For this review, take the finished solid that the model builds, in its own axes (mm). A direction names the side the tool comes from. Give positions to 0.01 mm unless a question says otherwise; leave off trailing zeros. Loops run counter-clockwise (first coordinate to the right, second up) from the corner with the lowest first, then second, coordinate; pieces in that order, holes last. Notation, with made-up numbers: (-22, -17.75) -> (-2, -17.75) arc R18 ccw to (-2, 9.25) -> close; hole circle Ø3 at (13.5, 10). An arc over 180 degrees is marked (long way). Write each question's results on one line, items separated by ' | '. Start each with the question number.
```python
from build123d import *

# Parameters (mm, degrees)
A_BASE_T42_OUTLINE_R               = 2.2479
A_BASE_T42_OUTLINE_R_2             = 1
A_BASE_T42_DEPTH                   = 3
OUTER_BRIM_DEPTH                   = 3
SKETCH5_W                          = 15
SKETCH5_H                          = 3
BASE_SUPPORTS_DEPTH                = 3
BASE_SUPPORTS_CHAMFER_SIZE         = 3
COVER_START                        = -3
SKETCH6_R                          = 1
COVER_DEPTH                        = 3
SKETCH2_W                          = 10.5
SKETCH2_H                          = 45
DYNAMIXEL_OFFSET_DEPTH             = 1.25
SKETCH3_W                          = 3
SKETCH3_H                          = 45
SKETCH3_H_2                        = 22.5
DYNAMIXEL_SIDE_SUPPORT_WALLS_DEPTH = 5.6
DYNAMIXEL_SUPPORT_CONTOURING_R     = 1


# Read off the part's stored shape, not the designer's step: a_base_t42
with BuildPart() as part:
    # a_base_t42 outline → a_base_t42 (new body)
    with BuildSketch(Plane(origin=(0, 0, 0), x_dir=(1, 0, 0), z_dir=(0, 1, 0))):
        with BuildLine():
            ThreePointArc((31.5, -42), (52.5, 0), (31.5, 42))
            Line((31.5, 42), (-31.5, 42))
            ThreePointArc((-31.5, 42), (-52.5, 0), (-31.5, -42))
            Line((-31.5, -42), (31.5, -42))
        make_face()
        with Locations((-23, -35)):
            Circle(A_BASE_T42_OUTLINE_R, mode=Mode.SUBTRACT)
        with Locations((23, -35)):
            Circle(A_BASE_T42_OUTLINE_R, mode=Mode.SUBTRACT)
        with Locations((-40.25, 0)):
            Circle(A_BASE_T42_OUTLINE_R_2, mode=Mode.SUBTRACT)
        with Locations((-23, 35)):
            Circle(A_BASE_T42_OUTLINE_R, mode=Mode.SUBTRACT)
        with Locations((40.25, 0)):
            Circle(A_BASE_T42_OUTLINE_R_2, mode=Mode.SUBTRACT)
        with Locations((23, 35)):
            Circle(A_BASE_T42_OUTLINE_R, mode=Mode.SUBTRACT)
    extrude(amount=A_BASE_T42_DEPTH)

    # Sketch1 → Outer Brim (add)
    with BuildSketch(Plane(origin=(0, 3, 0), x_dir=(1, 0, 0), z_dir=(0, 1, 0))):
        with BuildLine():
            Line((-31.5, -42), (31.5, -42))
            ThreePointArc((31.5, -42), (52.5, 0), (31.5, 42))
            Line((31.5, 42), (-31.5, 42))
            ThreePointArc((-31.5, 42), (-52.5, 0), (-31.5, -42))
        make_face()
        with BuildLine():
            Line((30.483602149, 39), (-30.483602149, 39))
            ThreePointArc((-30.483602149, 39), (-49.5, 0), (-30.483602149, -39))
            Line((-30.483602149, -39), (30.483602149, -39))
            ThreePointArc((30.483602149, -39), (49.5, 0), (30.483602149, 39))
        make_face(mode=Mode.SUBTRACT)
    extrude(amount=OUTER_BRIM_DEPTH)

    # Sketch5 → Base Supports (add)
    with BuildSketch(Plane(origin=(0, 3, 0), x_dir=(1, 0, 0), z_dir=(0, 1, 0))):
        with Locations((0, -27)):
            Rectangle(SKETCH5_W, SKETCH5_H)
        with Locations((0, 27)):
            Rectangle(SKETCH5_W, SKETCH5_H)
    extrude(amount=BASE_SUPPORTS_DEPTH)

    # Base Supports Chamfer
    base_supports_chamfer_edges = [part.edges().sort_by_distance(p)[0] for p in [
        (0, 3, 28.5),
        (0, 3, -28.5),
    ]]
    chamfer(base_supports_chamfer_edges, length=BASE_SUPPORTS_CHAMFER_SIZE - 0.0001)  # a hair under: the kernel refuses the full size

    # Sketch6 → Cover (add)
    with BuildSketch(Plane(origin=(0, 3, 0), x_dir=(1, 0, 0), z_dir=(0, 1, 0)).offset(COVER_START)):
        with Locations((-40.25, 0)):
            Circle(SKETCH6_R)
        with Locations((40.25, 0)):
            Circle(SKETCH6_R)
    extrude(amount=COVER_DEPTH)

    # Sketch2 → Dynamixel Offset (add)
    with BuildSketch(Plane(origin=(0, 3, 0), x_dir=(1, 0, 0), z_dir=(0, 1, 0))):
        with Locations((28.75, 0)):
            Rectangle(SKETCH2_W, SKETCH2_H)
        with Locations((-28.75, 0)):
            Rectangle(SKETCH2_W, SKETCH2_H)
    extrude(amount=DYNAMIXEL_OFFSET_DEPTH)

    # Sketch3 → Dynamixel Side Support Walls (add)
    with BuildSketch(Plane(origin=(0, 4.25, 0), x_dir=(1, 0, 0), z_dir=(0, 1, 0))):
        with Locations((-32.5, 0)):
            Rectangle(SKETCH3_W, SKETCH3_H)
        with Locations((-25, -11.25)):
            Rectangle(SKETCH3_W, SKETCH3_H_2)
        with Locations((25, 11.25)):
            Rectangle(SKETCH3_W, SKETCH3_H_2)
        with Locations((32.5, 0)):
            Rectangle(SKETCH3_W, SKETCH3_H)
    extrude(amount=DYNAMIXEL_SIDE_SUPPORT_WALLS_DEPTH)

    # Dynamixel Support Contouring
    dynamixel_support_contouring_edges = [part.edges().sort_by_distance(p)[0] for p in [
        (34, 6.425, -22.5),
        (23.5, 6.425, -22.5),
        (-23.5, 3.625, -22.5),
        (-34, 6.425, -22.5),
        (-34, 6.425, 22.5),
        (-23.5, 6.425, 22.5),
        (34, 6.425, 22.5),
        (23.5, 3.625, 22.5),
        (31, 9.85, 0),
        (26.5, 9.85, -11.25),
        (-26.5, 9.85, 11.25),
        (-31, 9.85, 0),
    ]]
    fillet(dynamixel_support_contouring_edges, radius=DYNAMIXEL_SUPPORT_CONTOURING_R)


solid = part.part
```
1. For pin 1 Ø2.5 at (y, z) = (6, -11) entering from +X; pin 2 Ø3.5 at (y, z) = (7, 10) entering from +X; pin 3 Ø5 at (x, z) = (-23, 35) entering from +Y, all flat-tipped, find the tip position at first contact; note any pin that passes through.
2. Machinability: for faces 1 (the flat face through (-34, 6, 0)), 2 (the cylindrical face through (-52.496, 2.958, -0.682)), which of the approach directions +Z, -Z, +X, -X, +Y, -Y give a long, thin tool a straight path to every point of the face, cutting with its end or side? Answer none if there is none.
3. We need section A-A (z = 35). Write out the cut boundary in (x, y).
4. Draft analysis for pull direction Z (two halves, no side actions). For faces 3 (the cylindrical face through (-49.496, 4.479, -0.629)), 4 (the flat face through (0, 6, -27)), 5 (the flat face through (0, 3, -42)), state which applies: released by +Z, released by -Z, zero draft, split by the parting line, or undercut.
5. Wall thickness on L1, parallel to X at y = 7.25, z = -8; L2, parallel to X at y = 7.5, z = 0.5; L3, parallel to Z at x = 23, y = 1.7: over which ranges is each line inside the solid? List them lowest first.
6. We need section C-C (z = 2). Write out the cut boundary in (x, y), plus the area to 3 significant figures.
7. We need section B-B (x = -45). Write out the cut boundary in (y, z), plus the area to 3 significant figures.
Response:
1) pin 1: stops at x = 51.59 | pin 2: stops at x = 51.8 | pin 3: stops at y = 3
2) face 1: +Y | face 2: -X, +Y, -Y
3) outline: (-39.13, 0) -> (-25.25, 0) -> (-25.25, 3) -> (-35, 3) -> (-35, 6) -> (-39.13, 6) -> close; (-20.75, 0) -> (20.75, 0) -> (20.75, 3) -> (-20.75, 3) -> close; (25.25, 0) -> (39.13, 0) -> (39.13, 6) -> (35, 6) -> (35, 3) -> (25.25, 3) -> close
4) face 3: undercut | face 4: zero draft | face 5: released by -Z
5) L1: x = -34 to -31, 23.5 to 26.5, 31 to 34 | L2: x = -34 to -31, -26.5 to -23.5, 31 to 34 | L3: z = -42 to -37.25, -32.75 to 32.75, 37.25 to 42
6) outline: (-52.46, 0) -> (52.46, 0) -> (52.46, 6) -> (49.46, 6) -> (49.46, 3) -> (34, 3) -> (34, 9.85) -> (32, 9.85) arc R1 ccw to (31, 8.85) -> (31, 4.25) -> (23.5, 4.25) -> (23.5, 3) -> (-23.5, 3) -> (-23.5, 9.85) -> (-25.5, 9.85) arc R1 ccw to (-26.5, 8.85) -> (-26.5, 4.25) -> (-31, 4.25) -> (-31, 8.85) arc R1 ccw to (-32, 9.85) -> (-34, 9.85) -> (-34, 3) -> (-49.46, 3) -> (-49.46, 6) -> (-52.46, 6) -> close | area: 409 mm2
7) outline: (0, -27.04) -> (6, -27.04) -> (6, -20.62) -> (3, -20.62) -> (3, 20.62) -> (6, 20.62) -> (6, 27.04) -> (0, 27.04) -> close | area: 201 mm2
